Design review of the part built by this model. Coordinates are the model's own, in mm. Face numbers are marked on the shaded views. A direction names the side the tool comes from. Give positions to 0.01 mm unless a question says otherwise; leave off trailing zeros. Order: outer loops, then holes, each group sorted by start corner. A loop starts at its lowest first (then second) coordinate and runs counter-clockwise, first axis right, second up.
```python
from build123d import *

# Parameters (mm, degrees)
BASE_SKETCH_W                   = 180
BASE_SKETCH_H                   = 180
BASE_EXTRUDE_DEPTH              = 20
SUPPORT_EXTRUDE_DEPTH           = 10
MOTOR_SUPPORT_SKETCH_R          = 90
MOTOR_SUPPORT_EXTRUDE_DEPTH     = 10
MOTOR_SKETCH_R                  = 65
MOTOR_EXTRUDE_DEPTH             = 180
MOTOR_EXTRUDE_DIRECTION_2_REACH = 249.184
MOTOR_HOLE_SKETCH_R             = 50
MOTOR_HOLE_CUT_DEPTH            = 210
SUPPORT_FILLETS_R               = 10


with BuildPart() as part:
    # Base Sketch → Base Extrude (new body)
    with BuildSketch(Plane.XY):
        Rectangle(BASE_SKETCH_W, BASE_SKETCH_H)
    extrude(amount=-BASE_EXTRUDE_DEPTH)

    # Support Sketch → Support Extrude (add)
    with BuildSketch(Plane(origin=(80, 0, 0), x_dir=(0, 0, -1), z_dir=(1, 0, 0))):
        Polygon((-100, 10), (-35, -55), (0, -55), (0, 70), (-100, 70), align=None)
    support_extrude = extrude(amount=-SUPPORT_EXTRUDE_DEPTH)

    # Support Mirror: Support Extrude across plane
    add(support_extrude.mirror(Plane(origin=(0, 0, 0), x_dir=(0, 0, 1), z_dir=(1, 0, 0))))

    # Motor Support Sketch → Motor Support Extrude (add)
    with BuildSketch(Plane(origin=(0, 50, 0), x_dir=(1, 0, 0), z_dir=(0, 1, 0))):
        with Locations((0, -100)):
            Circle(MOTOR_SUPPORT_SKETCH_R)
    extrude(amount=-MOTOR_SUPPORT_EXTRUDE_DEPTH)

    # Motor Sketch → Motor Extrude (add)
    with BuildSketch(Plane.XZ.offset(-40)):
        with Locations(Location((0, 100, 0), (0, 0, 90))):
            Circle(MOTOR_SKETCH_R)
    extrude(amount=MOTOR_EXTRUDE_DEPTH)

    # Motor Extrude direction 2: up to this face of the body (flat: up to its plane)
    motor_extrude_direction_2_end = Plane(part.part.faces().sort_by_distance((75, 70, 50))[0])
    # Motor Sketch → Motor Extrude direction 2 (add, up to the picked face)
    with BuildSketch(Plane.XZ.offset(-40), mode=Mode.PRIVATE) as motor_extrude_direction_2_sk1:
        with Locations(Location((0, 100, 0), (0, 0, 90))):
            Circle(MOTOR_SKETCH_R)
    motor_extrude_direction_2_tool1 = split(extrude(motor_extrude_direction_2_sk1.sketch, amount=-MOTOR_EXTRUDE_DIRECTION_2_REACH, mode=Mode.PRIVATE), bisect_by=motor_extrude_direction_2_end, keep=Keep.BOTH, mode=Mode.PRIVATE)
    add(motor_extrude_direction_2_tool1.solids().sort_by(Axis((0, 40, 100), (0, 1, 0)))[0])

    # Motor Hole Sketch → Motor Hole Cut (cut)
    with BuildSketch(Plane(origin=(0, 70, 0), x_dir=(1, 0, 0), z_dir=(0, 1, 0))):
        with Locations(Location((0, -100, 0), (0, 0, 270))):
            Circle(MOTOR_HOLE_SKETCH_R)
    extrude(amount=-MOTOR_HOLE_CUT_DEPTH, mode=Mode.SUBTRACT)

    # Support Fillets
    support_fillets_edges = [part.edges().sort_by_distance(p)[0] for p in [
        (75, 10, 100),
        (75, 70, 100),
        (70, 7.5, 0),
        (75, 70, 0),
        (75, -55, 0),
        (75, -55, 35),
        (80, 7.5, 0),
        (-75, 70, 100),
        (-75, 10, 100),
        (-75, -55, 35),
        (-80, 7.5, 0),
        (-75, -55, 0),
        (-75, 70, 0),
        (-70, 7.5, 0),
        (90, -90, -10),
        (-90, -90, -10),
        (-90, 90, -10),
        (90, 90, -10),
    ]]
    fillet(support_fillets_edges, radius=SUPPORT_FILLETS_R - 0.0001)  # a hair under: the kernel refuses the full size


solid = part.part
```
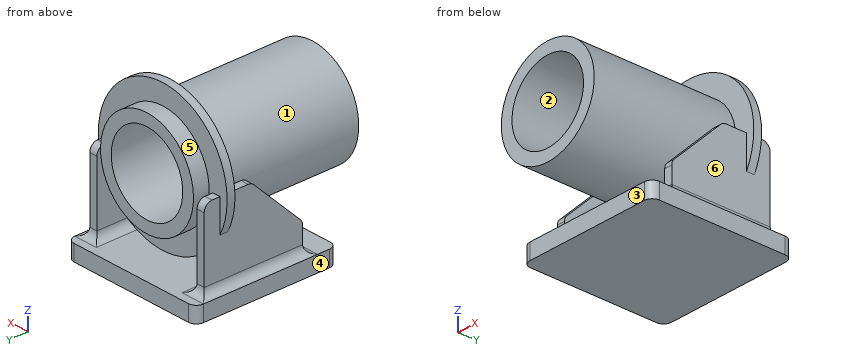
1. Draft analysis for pull direction X (two halves, no side actions). For the marked faces 4, 5 and 6, state which applies: pulls with the +X half, pulls with the -X half, needs draft (parallel to the pull), parting line crosses it, or undercut.
Recorded:
face 4: pulls with the -X half
face 5: undercut
face 6: pulls with the +X half
2. Take a section at D-D (y = -116). State the section outline as (x, z) points, then the cut area to 3 significant figures.
Recorded:
outline: circle Ø130 at (0, 100); hole circle Ø100 at (0, 100)
area: 5,420 mm2
3. Take a section at A-A (y = -46.5). State how many separate pieces and enclosed holes the cut face has, then the cut area to 3 significant figures.
Recorded:
separate pieces: 2
enclosed holes: 1
area: 9,980 mm2
4. Take a section at B-B (x = 0). State the section outline as (y, z) points.
Recorded:
outline: (-140, 35) - (40, 35) - (40, 10) - (50, 10) - (50, 35) - (70, 35) - (70, 50) - (-140, 50) - close; (-140, 150) - (70, 150) - (70, 165) - (50, 165) - (50, 190) - (40, 190) - (40, 165) - (-140, 165) - close; (-90, -20) - (90, -20) - (90, 0) - (-90, 0) - close
5. Machinability: for the marked faces 1, 2 and 3, which of the approach directions +Z, -Z, +X, -X, +Y, -Y give a long, thin tool a straight path to every point of the face, cutting with its end or side? Answer none if there is none.
Recorded:
face 1: -Y
face 2: +Y, -Y
face 3: -Z, +X, -X, -Y
6. For pin 1 (1.5 mm diameter, centred on x = -71.5, z = 78, fed in from -Y); pin 2 (11 mm diameter, centred on x = -74, y = 53, fed in from +Z); pin 3 (3 mm diameter, centred on x = -76.5, z = 17, fed in from -Y), all flat-tipped, find the tip position at first contact; note any pin that passes through.
Recorded:
pin 1: stops at y = -12.75
pin 2: stops at z = 157.31
pin 3: stops at y = -55
7. Take a section at C-C (z = 121). State the section outline as (x, y) points, then the cut area to 3 significant figures.
Recorded:
outline: (-87.52, 40) - (-61.51, 40) - (-61.51, -140) - (-45.38, -140) - (-45.38, 70) - (-61.51, 70) - (-61.51, 50) - (-87.52, 50) - close; (45.38, -140) - (61.51, -140) - (61.51, 40) - (87.52, 40) - (87.52, 50) - (61.51, 50) - (61.51, 70) - (45.38, 70) - close
area: 7,300 mm2
8. For line 1 along X through (y, z) = (-5, 100); line 2 along Z through (x, y) = (-44.5, -86.5); line 3 along Z through (x, y) = (-23.5, -80), list the stretches that pass through material, from the lowest coordinate up.
Recorded:
line 1: x = -65 to -50, 50 to 65
line 2: z = -20 to 0, 52.62 to 77.2, 122.8 to 147.38
line 3: z = -20 to 0, 39.4 to 55.87, 144.13 to 160.6
